The figure shows three views and two pictorial views of one solid part (mm, origin at its lowest corner). Answer the questions. Coordinates: 2 decimals unless noted, no trailing zeros. Order: outer loops, then holes, each group sorted by start corner. A loop starts at its lowest first (then second) coordinate and runs counter-clockwise, first axis right, second up. Notation, with made-up numbers: (70.5, -27) -> (95.5, -27) arc R26 cw to (95.5, -2) -> close; hole circle Ø5 at (36.5, 72.5). An arc over 180 degrees is marked (long way). Return JSON: item names as keys, results as strings.
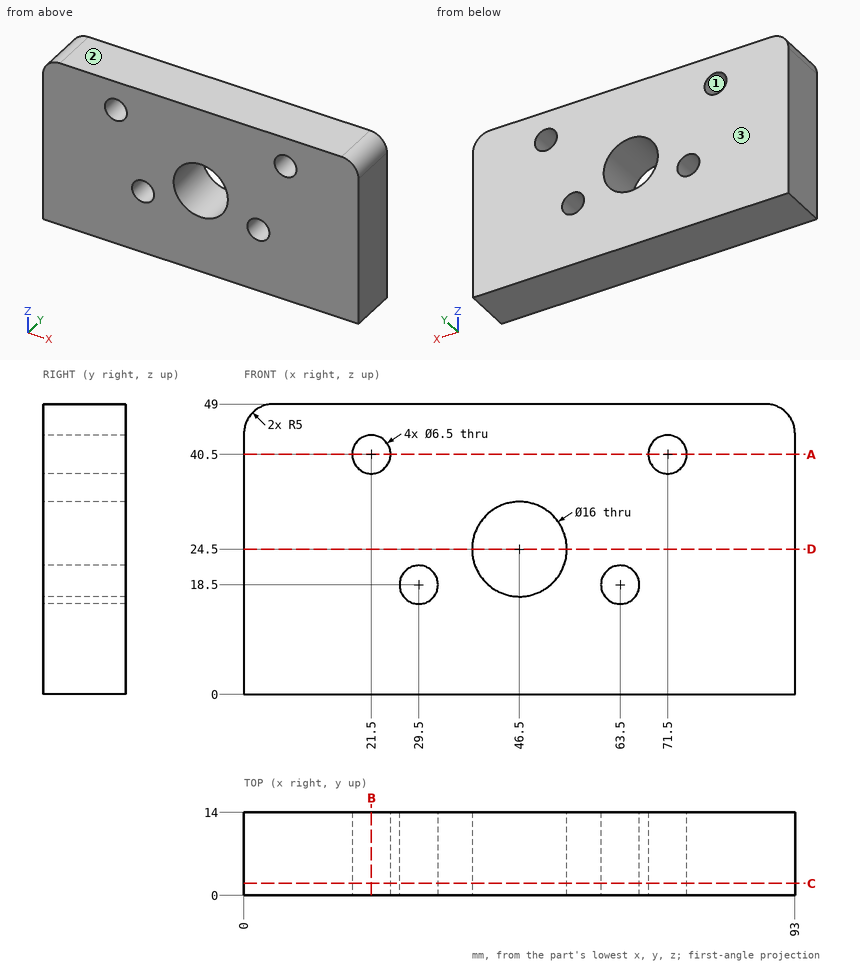
1. The part is cut by section A-A on z = 40.5. Give the vertices of the cut face in (x, y), and give its area (3 significant figures).
Answer block:
{"outline": "(0, 0) -> (18.25, 0) -> (18.25, 14) -> (0, 14) -> close; (24.75, 0) -> (68.25, 0) -> (68.25, 14) -> (24.75, 14) -> close; (74.75, 0) -> (93, 0) -> (93, 14) -> (74.75, 14) -> close", "area": "1,120 mm2"}
2. The part is cut by section D-D on z = 24.5. Give the vertices of the cut face in (x, y), and give its area (3 significant figures).
Answer block:
{"outline": "(0, 0) -> (38.5, 0) -> (38.5, 14) -> (0, 14) -> close; (54.5, 0) -> (93, 0) -> (93, 14) -> (54.5, 14) -> close", "area": "1,080 mm2"}
3. Consider line 1 (X direction, y = 6, z = 41); line 2 (Z direction, x = 29.5, y = 11.25); line 3 (X direction, y = 2.5, z = 42). Determine where each line is inside the solid, lowest interval first. Write a range as from..to.
Answer block:
{"line 1": "x = 0..18.29, 24.71..68.29, 74.71..93", "line 2": "z = 0..15.25, 21.75..49", "line 3": "x = 0..18.62, 24.38..68.62, 74.38..93"}
4. The part is cut by section B-B on x = 21.5. Give the vertices of the cut face in (y, z).
Answer block:
{"outline": "(0, 0) -> (14, 0) -> (14, 37.25) -> (0, 37.25) -> close; (0, 43.75) -> (14, 43.75) -> (14, 49) -> (0, 49) -> close"}
5. Determine the mould class of the marked faces 1, 2 and 3 for opening direction Z: pulls with the +Z half, pulls with the -Z half, needs draft (parallel to the pull), parting line crosses it, or undercut.
Answer block:
{"face 1": "undercut", "face 2": "pulls with the +Z half", "face 3": "needs draft"}
6. This flat-tipped pin is pushed along its axis until it touches: pin 1 Ø5 at (x, z) = (21.5, 40.5) entering from -Y. Where does it stop, or does it pass through?
Answer block:
{"pin 1": "passes through"}
7. The part is cut by section C-C on y = 2. Give the vertices of the cut face in (x, z).
Answer block:
{"outline": "(0, 0) -> (93, 0) -> (93, 44) arc R5 ccw to (88, 49) -> (5, 49) arc R5 ccw to (0, 44) -> close; hole circle Ø6.5 at (21.5, 40.5); hole circle Ø6.5 at (29.5, 18.5); hole circle Ø16 at (46.5, 24.5); hole circle Ø6.5 at (63.5, 18.5); hole circle Ø6.5 at (71.5, 40.5)"}
